Work out the finished part from the listing and answer in its coordinate system (mm). Face numbers are marked on the shaded views. A direction names the side the tool comes from. Round coordinates to 2 decimals unless told otherwise and drop trailing zeros. Loops run counter-clockwise (first coordinate to the right, second up) from the corner with the lowest first, then second, coordinate; pieces in that order, holes last. Notation, with made-up numbers: (53.5, 85.5) - (88.5, 85.5) arc R25 ccw to (88.5, 118.5) - close; hole circle Ø11 at (70.25, 3.5). An arc over 180 degrees is marked (long way). Answer as CSV lines item,"result". Start each with the question number.
Q1. Straight lines are drawn through the part: L1, parallel to Y at x = -121, z = 15.5; L2, parallel to X at y = 144, z = 7; L3, parallel to Y at x = -123, z = 14. For each, find the intervals that lie inside material, in ascending order. Write a range as [from, to].
Q2. Each of these flat-tipped pins is pushed along its axis until it touches: pin 1 Ø9 at (x, y) = (-120.83, 123.75) entering from +Z; pin 2 Ø5 at (x, z) = (-119.5, 4.5) entering from -Y; pin 3 Ø2 at (x, y) = (-122, 139) entering from -Z. Where does it stop, or does it pass through?
Q3. Section C-C on z = 14.25 is taken. Write down the section's boundary in (x, y), then the cut area to 3 significant figures.
Q4. The mould has two halves that part along Y. Classify the marked faces 1, 2 and 3: +Y half, -Y half, draft (parallel to the pull), parting line (faces both ways), or undercut.
Q5. Section D-D on y = 104.5 is taken. Write down the section's boundary in (x, z).
Q6. For the marked faces 4, 5 and 6, determine the directions among +Z, -Z, +X, -X, +Y, -Y from which every point of the face is accessible in a straight line to the end or side of a thin tool.
Q7. Section B-B on y = 114 is taken. Write down the section's boundary in (x, z), then the cut area to 3 significant figures.
```python
from build123d import *

# Parameters (mm, degrees)
SKETCH1_W                       = 16.5
SKETCH1_H                       = 66
BOSS_EXTRUDE1_DEPTH             = 20
SKETCH2_W                       = 16.5
SKETCH2_H                       = 33
SKETCH2_R                       = 5.85
SKETCH2_R_2                     = 5.05
CUT_EXTRUDE1_DEPTH              = 10
FILLET1_R                       = 10
FILLET2_R                       = 8.25
SKIZZE1_R                       = 5.1
AUFSATZ_LINEAR_AUSTRAGEN1_DEPTH = 7.3
SCHNITT_LINEAR_AUSTRAGEN1_DEPTH = 9


# Some blends are built 0.0001 mm under size
with BuildPart() as part:
    # Sketch1 → Boss-Extrude1 (new body)
    with BuildSketch(Plane.XY):
        with Locations((-120.834022786, 132)):
            Rectangle(SKETCH1_W, SKETCH1_H)
    extrude(amount=BOSS_EXTRUDE1_DEPTH)

    # Sketch2 → Cut-Extrude1 (cut)
    # profile 1 of 6: a face of its own
    with BuildSketch(Plane.XY.offset(20)):
        with Locations((-120.834022786, 115.5)):
            Rectangle(SKETCH2_W, SKETCH2_H)
        with Locations((-120.834022786, 107.25)):
            Circle(SKETCH2_R, mode=Mode.SUBTRACT)
        with Locations((-120.834022786, 123.75)):
            Circle(SKETCH2_R, mode=Mode.SUBTRACT)
    # profile 2 of 6: a face of its own
    with BuildSketch(Plane.XY.offset(20)):
        with Locations((-120.834022786, 148.5)):
            Rectangle(SKETCH2_W, SKETCH2_H)
        with Locations((-120.834022786, 140.25)):
            Circle(SKETCH2_R, mode=Mode.SUBTRACT)
        with Locations((-120.834022786, 156.75)):
            Circle(SKETCH2_R, mode=Mode.SUBTRACT)
    # profile 3 of 6: a face of its own
    with BuildSketch(Plane.XY.offset(20)):
        with Locations((-120.834022786, 140.25)):
            Circle(SKETCH2_R_2)
    # profile 4 of 6: a face of its own
    with BuildSketch(Plane.XY.offset(20)):
        with Locations((-120.834022786, 123.75)):
            Circle(SKETCH2_R_2)
    # profile 5 of 6: a face of its own
    with BuildSketch(Plane.XY.offset(20)):
        with Locations((-120.834022786, 107.25)):
            Circle(SKETCH2_R_2)
    # profile 6 of 6: a face of its own
    with BuildSketch(Plane.XY.offset(20)):
        with Locations((-120.834022786, 156.75)):
            Circle(SKETCH2_R_2)
    extrude(amount=-CUT_EXTRUDE1_DEPTH, mode=Mode.SUBTRACT)

    # Fillet1
    # the kernel refuses this fillet: 10 mm, written as the material it takes off along each edge
    with BuildSketch(Plane(origin=(-129.084022786, 165, -25), x_dir=(1, 0, 0), z_dir=(0, 0, 1))) as fillet1_piece_1:
        with BuildLine():
            CenterArc((FILLET1_R, -FILLET1_R), FILLET1_R, 90, 90)
            Line((0, -FILLET1_R), (0, 0))
            Line((0, 0), (FILLET1_R, 0))
        make_face()
    extrude(amount=60, mode=Mode.SUBTRACT)
    with BuildSketch(Plane(origin=(-112.584022786, 165, -25), x_dir=(-1, 0, 0), z_dir=(0, 0, 1))) as fillet1_piece_2:
        with BuildLine():
            CenterArc((FILLET1_R, FILLET1_R), FILLET1_R, 180, 90)
            Line((0, FILLET1_R), (0, 0))
            Line((0, 0), (FILLET1_R, 0))
        make_face()
    extrude(amount=60, mode=Mode.SUBTRACT)

    # Fillet2
    fillet2_edges = [part.edges().sort_by_distance(p)[0] for p in [
        (-129.084022786, 99, 5),
        (-112.584022786, 99, 5),
    ]]
    fillet(fillet2_edges, radius=FILLET2_R - 0.0001)  # a hair under: the kernel refuses the full size

    # Skizze1 → Aufsatz-Linear austragen1 (add)
    with BuildSketch(Plane.XY.offset(10)):
        with Locations((-120.834022786, 156.75)):
            Circle(SKIZZE1_R)
        with Locations((-120.834022786, 140.25)):
            Circle(SKIZZE1_R)
        with Locations((-120.834022786, 123.75)):
            Circle(SKIZZE1_R)
        with Locations((-120.834022786, 107.25)):
            Circle(SKIZZE1_R)
    extrude(amount=AUFSATZ_LINEAR_AUSTRAGEN1_DEPTH)

    # Skizze2 → Schnitt-Linear austragen1 (cut)
    with BuildSketch(Plane(origin=(0, 0, 0), x_dir=(-1, 0, 0), z_dir=(0, 0, -1))):
        with BuildLine():
            Line((127.084022786, 107.25), (127.084022786, 155))
            ThreePointArc((127.084022786, 155), (125.329020784, 160), (120.834022786, 162.806247498))
            ThreePointArc((120.834022786, 162.806247498), (116.339024787, 160), (114.584022786, 155))
            Line((114.584022786, 155), (114.584022786, 107.25))
            ThreePointArc((114.584022786, 107.25), (116.414605403, 102.830582618), (120.834022786, 101))
            ThreePointArc((120.834022786, 101), (125.253440168, 102.830582618), (127.084022786, 107.25))
        make_face()
    extrude(amount=-SCHNITT_LINEAR_AUSTRAGEN1_DEPTH, mode=Mode.SUBTRACT)


solid = part.part
```
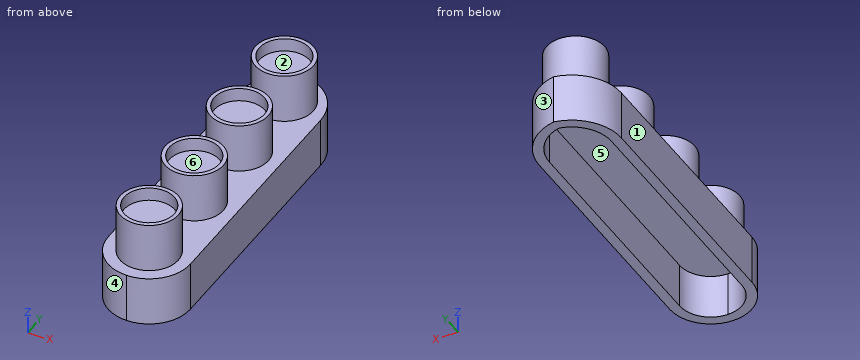
Findings:
1,L1,"y = [101.4, 113.1], [117.9, 129.6], [134.4, 146.1], [150.9, 162.6]"
1,L2,"x = [-129.08, -127.08], [-114.58, -112.58]"
1,L3,"y = [101.82, 112.68], [118.32, 129.18], [134.82, 145.68], [151.32, 162.18]"
2,pin 1,"stops at z = 17.3"
2,pin 2,"stops at y = 99"
2,pin 3,"stops at z = 9"
3,outline,"circle Ø11.7 at (-120.83, 107.25); circle Ø11.7 at (-120.83, 123.75); circle Ø11.7 at (-120.83, 140.25); circle Ø11.7 at (-120.83, 156.75)"
3,area,"430 mm^2"
4,face 1,"draft"
4,face 2,"undercut"
4,face 3,"+Y half"
5,outline,"(-128.61, 0) - (-126.45, 0) - (-126.45, 9) - (-115.22, 9) - (-115.22, 0) - (-113.06, 0) - (-113.06, 10) - (-115.67, 10) - (-115.67, 20) - (-116.6, 20) - (-116.6, 17.3) - (-125.07, 17.3) - (-125.07, 20) - (-126, 20) - (-126, 10) - (-128.61, 10) - close"
6,face 4,"+Z, -Z, -X, -Y"
6,face 5,"-Z"
6,face 6,"+Z"
7,outline,"(-129.08, 0) - (-127.08, 0) - (-127.08, 9) - (-114.58, 9) - (-114.58, 0) - (-112.58, 0) - (-112.58, 10) - (-129.08, 10) - close"
7,area,"52.5 mm^2"
